Study the drawing (mm; zero at the part's minimum x, y, z) and answer. Give positions to 0.01 mm unless a question says otherwise; leave off trailing zeros. Order: outer loops, then holes, each group sorted by start corner. A loop starts at its lowest first (then second) coordinate and runs counter-clockwise, first axis right, second up. Notation, with made-up numbers: (33, -28) - (86, -28) arc R18 ccw to (86, -1) - close; hole circle Ø6 at (1.25, 60). An arc over 180 degrees is marked (long way). Put each result on its own line as item: value.
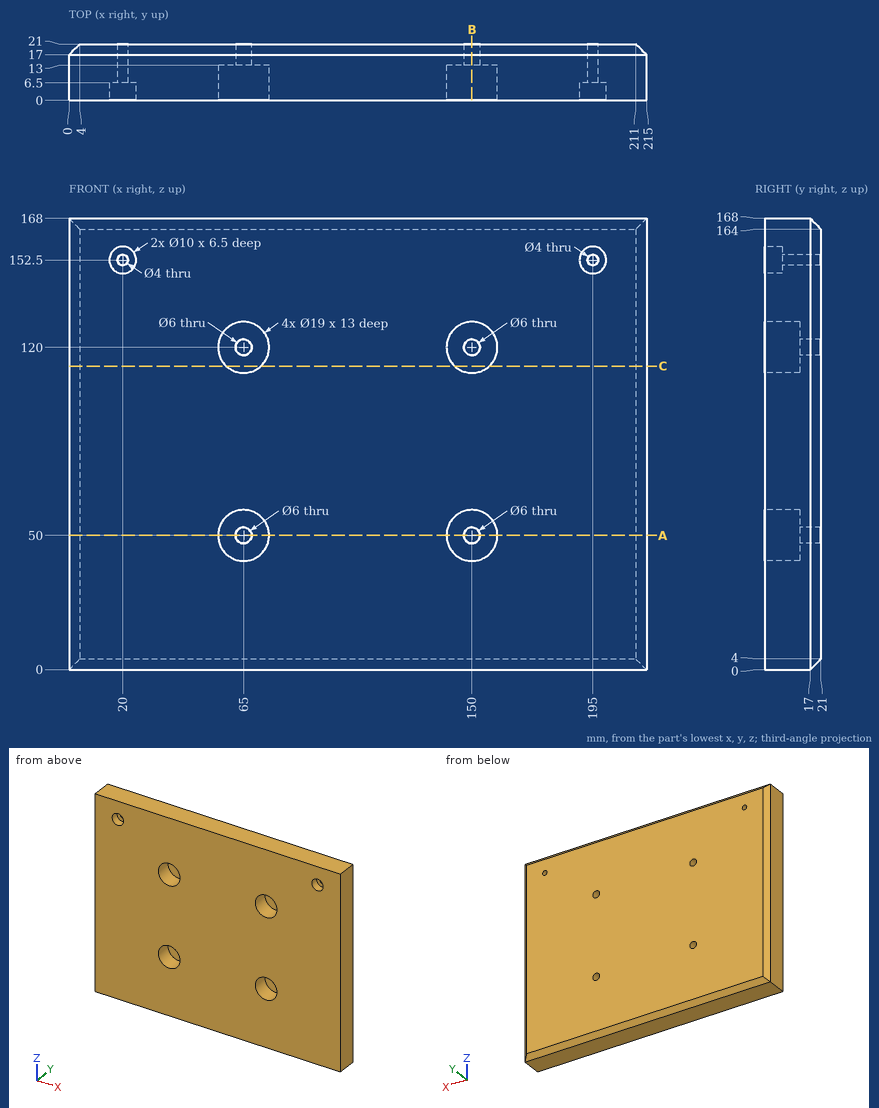
(1) Section C-C, the plane z = 113 is taken. Write down the section's boundary in (x, y), then the cut area to 3 significant figures.
Geometry check:
outline: (0, 0) - (58.58, 0) - (58.58, 13) - (71.42, 13) - (71.42, 0) - (143.58, 0) - (143.58, 13) - (156.42, 13) - (156.42, 0) - (215, 0) - (215, 17) - (211, 21) - (4, 21) - (0, 17) - close
area: 4,170 mm²
(2) Section A-A, the plane z = 50 is taken. Write down the section's boundary in (x, y).
Geometry check:
outline: (0, 0) - (55.5, 0) - (55.5, 13) - (62, 13) - (62, 21) - (4, 21) - (0, 17) - close; (68, 13) - (74.5, 13) - (74.5, 0) - (140.5, 0) - (140.5, 13) - (147, 13) - (147, 21) - (68, 21) - close; (153, 13) - (159.5, 13) - (159.5, 0) - (215, 0) - (215, 17) - (211, 21) - (153, 21) - close
(3) Given pin 1 (1.5 mm diameter, centred on y = 18, z = 103, fed in from -X); pin 2 (1 mm diameter, centred on x = 67.5, z = 117.5, fed in from -Y), each flat-ended and moving along its own axis, determine where each tip first touches the part or whether it passes through.
Geometry check:
pin 1: stops at x = 0.25
pin 2: stops at y = 13
(4) Straight lines are drawn through the part: line 1 (X direction, y = 9.5, z = 49.5); line 2 (Z direction, x = 65, y = 9.25); line 3 (X direction, y = 20, z = 52.5). For each, find the intervals that lie inside material, in ascending order.
Geometry check:
line 1: x = 0 to 55.51, 74.49 to 140.51, 159.49 to 215
line 2: z = 0 to 40.5, 59.5 to 110.5, 129.5 to 168
line 3: x = 3 to 63.34, 66.66 to 148.34, 151.66 to 212
(5) Section B-B, the plane x = 150 is taken. Write down the section's boundary in (y, z), then the cut area to 3 significant figures.
Geometry check:
outline: (0, 0) - (17, 0) - (21, 4) - (21, 47) - (13, 47) - (13, 40.5) - (0, 40.5) - close; (0, 59.5) - (13, 59.5) - (13, 53) - (21, 53) - (21, 117) - (13, 117) - (13, 110.5) - (0, 110.5) - close; (0, 129.5) - (13, 129.5) - (13, 123) - (21, 123) - (21, 164) - (17, 168) - (0, 168) - close
area: 2,920 mm²
